from build123d import *

# Parameters (mm, degrees)
F1_DEPTH = 6.096


with BuildPart() as f1:
    # F0 (on Front) → F1 (new body)
    with BuildSketch(Plane.XZ):
        with BuildLine():
            Line((-103.839319, 152.4), (-146.05, 152.4))
            ThreePointArc((-146.05, 152.4), (-150.540128, 150.540128), (-152.4, 146.05))
            Line((-152.4, 146.05), (-152.4, 3.175))
            ThreePointArc((-152.4, 3.175), (-151.470064, 0.929936), (-149.225, 0))
            Line((-149.225, 0), (-142.875, 0))
            ThreePointArc((-142.875, 0), (-140.629936, 0.929936), (-139.7, 3.175))
            Line((-139.7, 3.175), (-139.7, 76.2))
            ThreePointArc((-139.7, 76.2), (-138.770064, 78.445064), (-136.525, 79.375))
            ThreePointArc((-136.525, 79.375), (-134.279936, 78.445064), (-133.35, 76.2))
            Line((-133.35, 76.2), (-133.35, 3.175))
            ThreePointArc((-133.35, 3.175), (-132.420064, 0.929936), (-130.175, 0))
            Line((-130.175, 0), (-4.53437, 0))
            ThreePointArc((-4.53437, 0), (-1.933562, 1.353895), (-1.550846, 4.260914))
            Line((-1.550846, 4.260914), (-14.550568, 39.977357))
            ThreePointArc((-14.550568, 39.977357), (-20.654725, 42.823772), (-23.50114, 36.719615))
            Line((-23.50114, 36.719615), (-21.329312, 30.752567))
            ThreePointArc((-21.329312, 30.752567), (-21.435309, 28.32484), (-23.226922, 26.683129))
            Line((-23.226922, 26.683129), (-47.095115, 17.995817))
            ThreePointArc((-47.095115, 17.995817), (-49.522842, 18.101814), (-51.164553, 19.893427))
            Line((-51.164553, 19.893427), (-97.872271, 148.221828))
            ThreePointArc((-97.872271, 148.221828), (-100.197109, 151.251615), (-103.839319, 152.4))
        make_face()
    extrude(amount=-F1_DEPTH)


solid = f1.part
Read the model definition and answer for the solid it produces. Units are mm, in the model's axes. A direction names the side the tool comes from. Round coordinates to 2 decimals unless told otherwise and drop trailing zeros. Order: outer loops, then holes, each group sorted by start corner. A loop starts at its lowest first (then second) coordinate and runs counter-clockwise, first axis right, second up.
1) The mould has two halves that part along X. Classify faces 1 (the face through (-139.7, 3, 39)), 2 (the face through (-152.4, 3, 76)), 3 (the face through (-68, 3, 0)): released by +X, released by -X, zero draft, split by the parting line, or undercut.
2) The part is cut by section A-A on z = 48.5. Write down the section's boundary in (x, y).
3) Straight lines are drawn through the part: L1, parallel to X at y = 4.25, z = 40.5; L2, parallel to X at y = 2.25, z = 30; L3, parallel to X at y = 4.75, z = 45. For each, find the intervals that lie inside material, in ascending order.
4) The part is cut by section C-C on x = -11.5. Write down the section's boundary in (y, z), plus the area to 3 significant figures.
5) Flat-ended cylindrical pins translate along their axes: pin 1 (1 mm diameter, centred on y = 1.5, z = 19.5, fed in from +X); pin 2 (1.8 mm diameter, centred on y = 1.5, z = 48, fed in from +X). Find the tip coordinate at first contact, or state that the pin passes through.
6) The part is cut by section D-D on z = 11. Write down the section's boundary in (x, y), plus the area to 3 significant figures.
7) For faces 4 (the face through (-133.35, 3, 40)), 5 (the face through (-74.19, 3.01, 83.16)), 6 (the face through (-125, 3, 152.4)), 7 (the face through (-21.4, 3, 28.4)), determine the directions among +Z, -Z, +X, -X, +Y, -Y from which every point of the face is accessible in a straight line to the end or side of a thin tool.
Resolved:
1. face 1: undercut
1. face 2: released by -X
1. face 3: zero draft
2. outline: (-152.4, 0) - (-139.7, 0) - (-139.7, 6.1) - (-152.4, 6.1) - close; (-133.35, 0) - (-61.58, 0) - (-61.58, 6.1) - (-133.35, 6.1) - close
3. L1: x = -152.4 to -139.7, -133.35 to -58.66, -23.27 to -14.78
3. L2: x = -152.4 to -139.7, -133.35 to -54.84, -21.16 to -10.92
3. L3: x = -152.4 to -139.7, -133.35 to -60.3
4. outline: (0, 0) - (6.1, 0) - (6.1, 31.6) - (0, 31.6) - close
4. area: 193 mm2
5. pin 1: stops at x = -6.92
5. pin 2: stops at x = -61.07
6. outline: (-152.4, 0) - (-139.7, 0) - (-139.7, 6.1) - (-152.4, 6.1) - close; (-133.35, 0) - (-4, 0) - (-4, 6.1) - (-133.35, 6.1) - close
6. area: 866 mm2
7. face 4: -Z, +Y, -Y
7. face 5: +Z, +Y, -Y
7. face 6: +Z, +X, -X, +Y, -Y
7. face 7: +Y, -Y
